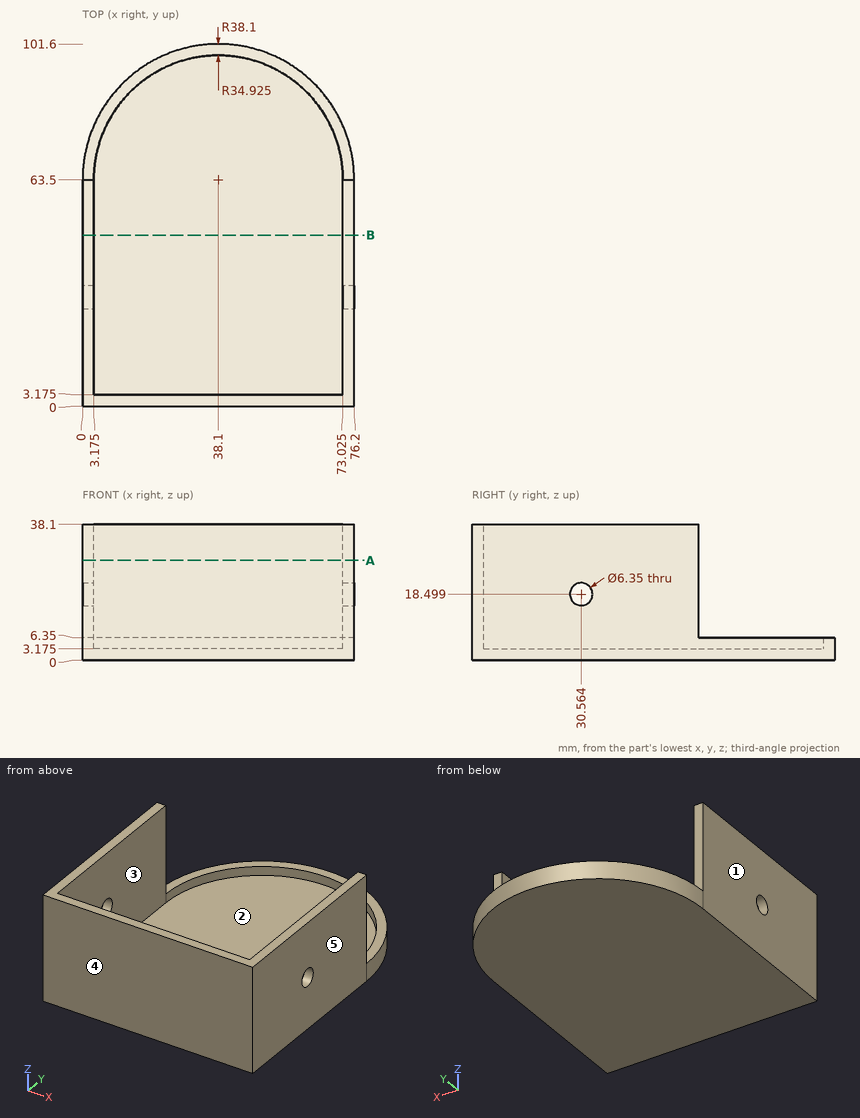
Study the drawing (mm; zero at the part's minimum x, y, z) and answer. A direction names the side the tool comes from. Give positions to 0.01 mm unless a question says otherwise; leave off trailing zeros. Loops run counter-clockwise (first coordinate to the right, second up) from the corner with the lowest first, then second, coordinate; pieces in that order, holes last. Notation, with made-up numbers: (-30.75, 2) - (-21.75, 2) arc R14 cw to (-21.75, 6) - close; hole circle Ø3 at (-8.5, 89.5). An arc over 180 degrees is marked (long way). Return JSON: item names as keys, results as strings. Group by question number.
1. Find section B-B (y = 48). Write down the section's boundary in (x, z) (1 decimal).
2. Given pin 1 Ø2.5 at (x, z) = (1, 30) entering from +Y; pin 2 Ø3 at (x, z) = (35.5, 19.5) entering from +Y (3 decimals); pin 3 Ø4 at (x, y) = (63.5, 16.5) entering from +Z (3 decimals); pin 4 Ø4 at (y, z) = (30.56, 18.5) entering from +X, each flat-ended and moving along its own axis, determine where each tip first touches the part or whether it passes through.
3. Find section A-A (z = 28). Write down the section's boundary in (x, y) (1 decimal).
4. Which of the six approach directions +Z, -Z, +X, -X, +Y, -Y give full straight-line access (tool end or side, diameter ignored) to the marked faces 1 and 2?
5. Determine the mould class of the marked faces 3, 4 and 5 for opening direction X: pulls with the +X half, pulls with the -X half, needs draft (parallel to the pull), parting line crosses it, or undercut.
6. Straight lines are drawn through the part: line 1 (X direction, y = 9, z = 27.5) (1 decimal); line 2 (Y direction, x = 41, z = 24.5) (1 decimal). For each, find the intervals that lie inside material, in ascending order. Write a range as [from, to].
Verdict:
{
 "1": {"outline": "(0, 0) - (76.2, 0) - (76.2, 38.1) - (73, 38.1) - (73, 3.2) - (3.2, 3.2) - (3.2, 38.1) - (0, 38.1) - close"},
 "2": {"pin 1": "stops at y = 63.5", "pin 2": "stops at y = 3.175", "pin 3": "stops at z = 3.175", "pin 4": "passes through"},
 "3": {"outline": "(0, 0) - (76.2, 0) - (76.2, 63.5) - (73, 63.5) - (73, 3.2) - (3.2, 3.2) - (3.2, 63.5) - (0, 63.5) - close"},
 "4": {"face 1": "+Z, -Z, -X, +Y, -Y", "face 2": "+Z"},
 "5": {"face 3": "undercut", "face 4": "needs draft", "face 5": "pulls with the +X half"},
 "6": {"line 1": "x = [0, 3.2], [73, 76.2]", "line 2": "y = [0, 3.2]"}
}
